Geometry: final body of the model. Coordinates: model frame, mm. Give positions to 0.01 mm unless a question says otherwise; leave off trailing zeros. Order: outer loops, then holes, each group sorted by start corner. A loop starts at its lowest first (then second) coordinate and runs counter-clockwise, first axis right, second up. Notation, with made-up numbers: (-28.5, -11) -> (-19.5, -11) arc R25 cw to (-19.5, 6) -> close; hole circle Ø6 at (-19, -9). An arc over 180 degrees is marked (long way). Write item = value, one per line.
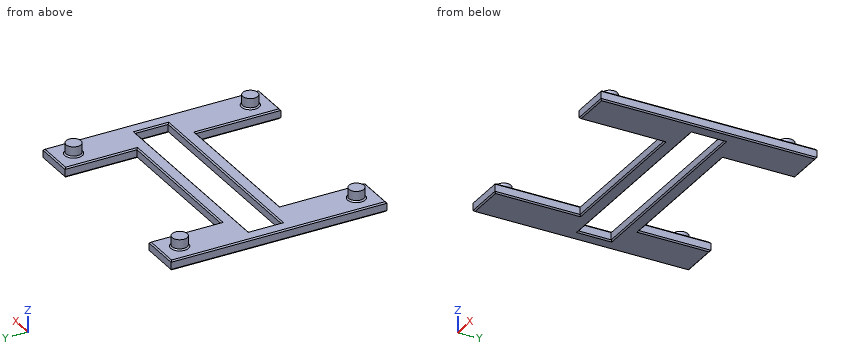
```python
from build123d import *

# Parameters (mm, degrees)
SKETCH_W        = 31
SKETCH_H        = 5
PAD_DEPTH       = 1.5
SKETCH001_R     = 1.15
PAD001_DEPTH    = 1.6
CHAMFER_SIZE    = 0.2
CHAMFER001_SIZE = 0.2


with BuildPart() as part:
    # Sketch → Pad (new body)
    with BuildSketch(Plane.XY):
        Polygon((35, 0), (35, 33), (29, 33), (29, 22), (6, 22), (6, 33), (0, 33), (0, 0), (6, 0), (6, 13), (29, 13), (29, 0), align=None)
        with Locations((17.5, 17.5)):
            Rectangle(SKETCH_W, SKETCH_H, mode=Mode.SUBTRACT)
    extrude(amount=PAD_DEPTH)

    # Sketch001 → Pad001 (new body)
    with BuildSketch(Plane.XY.offset(1.5)):
        with Locations((3, 30)):
            Circle(SKETCH001_R)
        with Locations((32, 30)):
            Circle(SKETCH001_R)
        with Locations((32, 3)):
            Circle(SKETCH001_R)
        with Locations((3, 3)):
            Circle(SKETCH001_R)
    extrude(amount=PAD001_DEPTH)

    # Chamfer
    chamfer_edges = [part.edges().sort_by_distance(p)[0] for p in [
        (0, 16.5, 1.5),
        (3, 33, 1.5),
        (3, 0, 1.5),
        (6, 27.5, 1.5),
        (6, 6.5, 1.5),
        (17.5, 22, 1.5),
        (17.5, 13, 1.5),
        (29, 27.5, 1.5),
        (29, 6.5, 1.5),
        (32, 33, 1.5),
        (32, 0, 1.5),
        (35, 16.5, 1.5),
        (1.85, 3, 1.5),
        (30.85, 3, 1.5),
        (1.85, 30, 1.5),
        (30.85, 30, 1.5),
        (2, 17.5, 1.5),
        (17.5, 20, 1.5),
        (17.5, 15, 1.5),
        (33, 17.5, 1.5),
    ]]
    chamfer(chamfer_edges, length=CHAMFER_SIZE)

    # Chamfer001
    chamfer001_edges = [part.edges().sort_by_distance(p)[0] for p in [
        (0, 16.5, 0),
        (3, 0, 0),
        (6, 6.5, 0),
        (17.5, 13, 0),
        (29, 6.5, 0),
        (32, 0, 0),
        (35, 16.5, 0),
        (32, 33, 0),
        (29, 27.5, 0),
        (17.5, 22, 0),
        (6, 27.5, 0),
        (3, 33, 0),
        (2, 17.5, 0),
        (17.5, 20, 0),
        (33, 17.5, 0),
        (17.5, 15, 0),
    ]]
    chamfer(chamfer001_edges, length=CHAMFER001_SIZE)


solid = part.part
```
1) Section query C-C (x = 3). Output: boundary loops of the cut face in (y, z).
Check sheet entries:
outline = (0, 0.2) -> (0.2, 0) -> (14.8, 0) -> (15, 0.2) -> (15, 1.3) -> (14.8, 1.5) -> (4.35, 1.5) -> (4.15, 1.7) -> (4.15, 3.1) -> (1.85, 3.1) -> (1.85, 1.7) -> (1.65, 1.5) -> (0.2, 1.5) -> (0, 1.3) -> close; (20, 0.2) -> (20.2, 0) -> (32.8, 0) -> (33, 0.2) -> (33, 1.3) -> (32.8, 1.5) -> (31.35, 1.5) -> (31.15, 1.7) -> (31.15, 3.1) -> (28.85, 3.1) -> (28.85, 1.7) -> (28.65, 1.5) -> (20.2, 1.5) -> (20, 1.3) -> close
2) Line query: line 1 (X direction, y = 17, z = 0.3); line 2 (Y direction, x = 32, z = 2.55); line 3 (X direction, y = 4, z = 1.3). Output: solid intervals per line, ascending. Write a range as from..to.
Check sheet entries:
line_1 = 0..2, 33..35
line_2 = 1.85..4.15, 28.85..31.15
line_3 = 0..6, 29..35
3) Section query A-A (y = 30). Output: boundary loops of the cut face in (x, z).
Check sheet entries:
outline = (0, 0.2) -> (0.2, 0) -> (5.8, 0) -> (6, 0.2) -> (6, 1.3) -> (5.8, 1.5) -> (4.35, 1.5) -> (4.15, 1.7) -> (4.15, 3.1) -> (1.85, 3.1) -> (1.85, 1.7) -> (1.65, 1.5) -> (0.2, 1.5) -> (0, 1.3) -> close; (29, 0.2) -> (29.2, 0) -> (34.8, 0) -> (35, 0.2) -> (35, 1.3) -> (34.8, 1.5) -> (33.35, 1.5) -> (33.15, 1.7) -> (33.15, 3.1) -> (30.85, 3.1) -> (30.85, 1.7) -> (30.65, 1.5) -> (29.2, 1.5) -> (29, 1.3) -> close
4) Section query B-B (x = 7). Output: boundary loops of the cut face in (y, z), plus the area to 3 significant figures.
Check sheet entries:
outline = (13, 0.2) -> (13.2, 0) -> (14.8, 0) -> (15, 0.2) -> (15, 1.3) -> (14.8, 1.5) -> (13.2, 1.5) -> (13, 1.3) -> close; (20, 0.2) -> (20.2, 0) -> (21.8, 0) -> (22, 0.2) -> (22, 1.3) -> (21.8, 1.5) -> (20.2, 1.5) -> (20, 1.3) -> close
area = 5.84 mm²
5) First-contact query: P1, Ø1.2, axis at x = 22, z = 0.5, coming from the +Y side; P2, Ø0.6, axis at x = 16, z = 0.5, coming from the -Y side; P3, Ø16.5, axis at x = 15, y = 11, coming from the +Z side. Flat tips, straight axial feed; report the tip coordinate or a pass-through.
Check sheet entries:
P1 = 22
P2 = 13
P3 = 1.5
6) Section query D-D (y = 5.5). Output: boundary loops of the cut face in (x, z).
Check sheet entries:
outline = (0, 0.2) -> (0.2, 0) -> (5.8, 0) -> (6, 0.2) -> (6, 1.3) -> (5.8, 1.5) -> (0.2, 1.5) -> (0, 1.3) -> close; (29, 0.2) -> (29.2, 0) -> (34.8, 0) -> (35, 0.2) -> (35, 1.3) -> (34.8, 1.5) -> (29.2, 1.5) -> (29, 1.3) -> close
